CAD build for the part. Positions are in the model's coordinates, mm. Round coordinates to 2 decimals unless told otherwise and drop trailing zeros. Loops run counter-clockwise (first coordinate to the right, second up) from the corner with the lowest first, then second, coordinate; pieces in that order, holes last. Notation, with made-up numbers: M 50.25,12.5 L 68.25,12.5 A10 cw 68.25,25.5 Z; hole C -5,43.25 d11. An arc over 180 degrees is marked long. Use one line per item in the form item = value.
Autodesk Inventor part; units mm, degrees
ref_plane "Work Plane1" through (-7.9612, 0, 0) normal (0, -0.866, -0.5) x (1, 0, 0)
ref_plane "YZ Plane" through (0, 0, 0) normal (1, 0, 0) x (0, 1, 0)
ref_plane "XZ Plane" through (0, 0, 0) normal (0, 1, 0) x (-1, 0, 0)
sketch "Boceto1" plane through (0, 0, 0) normal (1, 0, 0) x (0, 1, 0)
  line L0 (-4.0415, 0) -> (-2.0207, 3.5)
  line L1 (-2.0207, 3.5) -> (2.0207, 3.5)
  line L2 (2.0207, 3.5) -> (4.0415, 0)
  line L3 (4.0415, 0) -> (2.0207, -3.5)
  line L4 (2.0207, -3.5) -> (-2.0207, -3.5)
  line L5 (-2.0207, -3.5) -> (-4.0415, 0)
  point P0 (0, 0)
  point P1 (0, 0)
  dimension "d0" = 8.0829
extrude "Cuerpo" add sketch "Boceto1" along normal blind 3.2
sketch "Boceto2" plane through (0, 0, 0) normal (0, 0, 1) x (1, 0, 0)
  line L0 (0, 2.0207) -> (0, 4.0415)
  line L1 (0, 4.0415) -> (3.2, 4.0415)
  line L2 (3.2, 2.0207) -> (3.2, 4.0415)
  line L3 (-0.64, 0) -> (3.84, 0)
  line L4 (0.3126, 4.0415) -> (0, 3.5)
  line L5 (2.8874, 4.0415) -> (3.2, 3.5)
  dimension "d3" = 30
  dimension "d4" = 30
  dimension "d5" = 7
  dimension "d6" = 7
revolve "Chaflán1" cut sketch "Boceto2" angle 360 about axis through (-10, 0, 0) along (1, 0, 0)
sketch "Boceto3" plane through (3.2, 0, 0) normal (1, 0, 0) x (0, 0, -1)
  arc A0 (-1.75, -3.0311) -> (1.75, -3.0311) centre (0, 0) ccw
hole "Rosca" at (3.2, 0, 0) direction (-1, 0, 0) diameter 3.242 end through all
chamfer "Chaflán2" distance 0.3789 angle 30 1 edges at (3.2, 0, 1.621) measured on face at (3.2, 2.8569, -0.0651)
chamfer "Chaflán3" distance 0.3789 angle 30 1 edges at (0, 0, 1.621) measured on face at (0, 2.8569, -0.0651)
ref_plane "Work Plane1" through (-7.9612, 0, 0) normal (0, -0.866, -0.5) x (1, 0, 0)
equation "\"d0\" = 1.1547 * SW"
equation "\"d1\" = KOH"
equation "\"d3\" = ANG1"
equation "\"d4\" = ANG2"
equation "\"d5\" = SW0"
equation "\"d6\" = SW01"
equation "\"d8\" = -0.5 * GD1 + 0.5 * NND"
equation "\"d40\" = -0.5 * GD1 + 0.5 * NND"
equation "\"d10\" = -0.5 * GD1 + 0.5 * NND"
equation "\"d41\" = -0.5 * GD1 + 0.5 * NND"
equation "\"ANG1\" = 30deg"
equation "\"ANG2\" = 30deg"
equation "\"NND\" = 4"
equation "\"KOH\" = 3.2"
equation "\"SW\" = 7"
equation "\"SW0\" = SW"
equation "\"SW01\" = SW"
equation "\"GUL\" = 0.541266 * PTC"
equation "\"WFT\" = 0.4"
equation "\"THREADDIA\" = 4"
equation "\"TOA\" = 30deg"
equation "\"PTC\" = 0.7"
equation "\"E0\" = 1.155 * SW"
equation "\"GAL\" = 0.541266 * PTC"
properties part number "AS 1112 - M4  Tipo 5" material "Acero, suave"
1. Cut at A-A on x = 1.25. Write the cut outline in (y, z), and give its area (3 significant figures).
Completed:
outline = M -4.04,0 L -2.02,-3.5 L 2.02,-3.5 L 4.04,0 L 2.02,3.5 L -2.02,3.5 Z; hole C 0,0 d3.24
area = 34.2 mm2
2. Pull direction Y, two halves, no side cores. Call faces 1 (the face through (1.581, 1.438, -0.748)), 2 (the face through (1.578, -3.045, 1.726)), 3 (the face through (3.124, 1.808, 3.15)): +Y half, -Y half, draft (parallel to the pull), parting line (faces both ways), or undercut.
Completed:
face_1 = undercut
face_2 = -Y half
face_3 = +Y half
3. Probe line 1 along Z through (x, y) = (2.1, 0); line 2 along Z through (x, y) = (2.3, 0.75); line 3 along Y through (x, z) = (0.75, -0.75). List the from-to ranges inside material, lowest first. Write a range as from..to.
Completed:
line_1 = -3.5..-1.62, 1.62..3.5
line_2 = -3.5..-1.44, 1.44..3.5
line_3 = -3.61..-1.44, 1.44..3.61
4. Drop a flat-ended pin along its axis: P1, Ø1.9, axis at y = 0, z = 0, coming from the +X side. Give the stop position or say it passes through.
Completed:
P1 = through
